Part model, mm, in its own coordinate system. Face numbers are marked on the shaded views. A direction names the side the tool comes from. Coordinates: 2 decimals unless noted, no trailing zeros. Loops run counter-clockwise (first coordinate to the right, second up) from the corner with the lowest first, then second, coordinate; pieces in that order, holes last. Notation, with made-up numbers: (88.25, 59.5) -> (134.25, 59.5) arc R23 ccw to (134.25, 87.5) -> close; hole circle Ø5 at (32.25, 29). An arc over 180 degrees is marked (long way). One line per question, with ' | ' between items. Start each with the question number.
1) Cut at C-C (y = -0.5). List the corners of the cut face in (x, z) (3 decimals), plus the area to 3 significant figures.
2) 3-axis set-ups, long thin cutter, end or side, ignore diameter. For the marked faces 4, 5, 6 and 7: which of +Z, -Z, +X, -X, +Y, -Y reach the whole face in a straight line?
3) Two-plate mould, pull along X, no slides. Class the marked faces 1, 2 and 3: released by +X, released by -X, zero draft, split by the parting line, or undercut.
4) Cut at D-D (z = 0.8). List the corners of the cut face in (x, y) (3 decimals), plus the area to 3 significant figures.
5) Drop flat-ended pins along their axis: pin 1 (1.2 mm diameter, centred on x = -3.5, y = 0, fed in from +Z); pin 2 (1.4 mm diameter, centred on x = -7, z = -0.5, fed in from -Y); pin 3 (1.4 mm diameter, centred on x = -7, z = -0.5, fed in from +Y). Give the stop position or say it passes through.
6) Cut at B-B (y = 1.1). List the corners of the cut face in (x, z) (3 decimals), plus the area to 3 significant figures.
7) Cut at A-A (x = 0). List the corners of the cut face in (y, z) (3 decimals), plus the area to 3 significant figures.
8) Probe L1, parallel to Z at x = 0, y = -0.7; L2, parallel to Y at x = -7.5, z = -0.35; L3, parallel to Z at x = -3.25, y = -0.6. List the from-to ranges inside material, lowest first. Write a range as from..to.
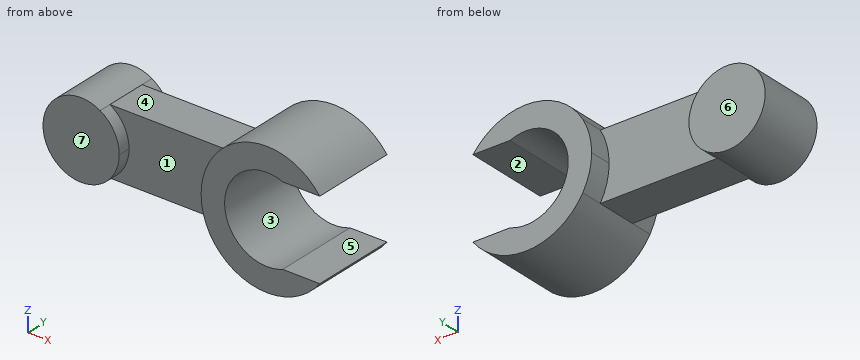
from build123d import *

# Parameters (mm, degrees)
F1_DEPTH = 1.23
F2_DEPTH = 0.765
F3_DEPTH = 1.595
F4_DEPTH = 1.595
F5_DEPTH = 0.765
F6_DEPTH = 1.23


with BuildPart() as f1:
    # F0 (on Front) → F1 (new body)
    with BuildSketch(Plane.XZ):
        with BuildLine():
            ThreePointArc((-6.54775, -1.24), (-6.022378, -0.716374), (-5.83, 0))
            ThreePointArc((-5.83, 0), (-6.022378, 0.716374), (-6.54775, 1.24))
            ThreePointArc((-6.54775, 1.24), (-8.69, 0), (-6.54775, -1.24))
        make_face()
    extrude(amount=F1_DEPTH)

    # F0 (on Front) → F2 (join)
    with BuildSketch(Plane.XZ):
        with BuildLine():
            Line((-5.83, 0), (-5.83, 1.24))
            Line((-5.83, 1.24), (-6.54775, 1.24))
            ThreePointArc((-6.54775, 1.24), (-6.022378, 0.716374), (-5.83, 0))
        make_face()
        with BuildLine():
            Line((-6.54775, -1.24), (-5.83, -1.24))
            Line((-5.83, -1.24), (-5.83, 0))
            ThreePointArc((-5.83, 0), (-6.022378, -0.716374), (-6.54775, -1.24))
        make_face()
        with BuildLine():
            ThreePointArc((-2.47, 0), (-2.385088, 0.642073), (-2.136188, 1.24))
            Line((-2.136188, 1.24), (-5.83, 1.24))
            Line((-5.83, 1.24), (-5.83, 0))
            Line((-5.83, 0), (-2.47, 0))
        make_face()
        with BuildLine():
            Line((-5.83, -1.24), (-2.136188, -1.24))
            ThreePointArc((-2.136188, -1.24), (-2.385088, -0.642073), (-2.47, 0))
            Line((-2.47, 0), (-5.83, 0))
            Line((-5.83, 0), (-5.83, -1.24))
        make_face()
    extrude(amount=F2_DEPTH)

    # F0 (on Front) → F3 (join)
    with BuildSketch(Plane.XZ):
        with BuildLine():
            Line((1.7075, 1.475), (1.981231, 1.475))
            ThreePointArc((1.981231, 1.475), (-0.140745, 2.465987), (-2.136188, 1.24))
            ThreePointArc((-2.136188, 1.24), (-2.385088, 0.642073), (-2.47, 0))
            ThreePointArc((-2.47, 0), (-2.385088, -0.642073), (-2.136188, -1.24))
            ThreePointArc((-2.136188, -1.24), (-0.140745, -2.465987), (1.981231, -1.475))
            Line((1.981231, -1.475), (1.7075, -1.475))
            Line((1.7075, -1.475), (0.593696, -1.475))
            ThreePointArc((0.593696, -1.475), (-1.59, 0), (0.593696, 1.475))
            Line((0.593696, 1.475), (1.7075, 1.475))
        make_face()
    extrude(amount=F3_DEPTH)

    # F0 (on Front) → F4 (join)
    with BuildSketch(Plane.XZ):
        with BuildLine():
            Line((1.7075, 1.475), (1.981231, 1.475))
            ThreePointArc((1.981231, 1.475), (-0.140745, 2.465987), (-2.136188, 1.24))
            ThreePointArc((-2.136188, 1.24), (-2.385088, 0.642073), (-2.47, 0))
            ThreePointArc((-2.47, 0), (-2.385088, -0.642073), (-2.136188, -1.24))
            ThreePointArc((-2.136188, -1.24), (-0.140745, -2.465987), (1.981231, -1.475))
            Line((1.981231, -1.475), (1.7075, -1.475))
            Line((1.7075, -1.475), (0.593696, -1.475))
            ThreePointArc((0.593696, -1.475), (-1.59, 0), (0.593696, 1.475))
            Line((0.593696, 1.475), (1.7075, 1.475))
        make_face()
    extrude(amount=-F4_DEPTH)

    # F0 (on Front) → F5 (join)
    with BuildSketch(Plane.XZ):
        with BuildLine():
            Line((-6.54775, -1.24), (-5.83, -1.24))
            Line((-5.83, -1.24), (-5.83, 0))
            ThreePointArc((-5.83, 0), (-6.022378, -0.716374), (-6.54775, -1.24))
        make_face()
        with BuildLine():
            Line((-5.83, 0), (-5.83, 1.24))
            Line((-5.83, 1.24), (-6.54775, 1.24))
            ThreePointArc((-6.54775, 1.24), (-6.022378, 0.716374), (-5.83, 0))
        make_face()
        with BuildLine():
            ThreePointArc((-2.47, 0), (-2.385088, 0.642073), (-2.136188, 1.24))
            Line((-2.136188, 1.24), (-5.83, 1.24))
            Line((-5.83, 1.24), (-5.83, 0))
            Line((-5.83, 0), (-2.47, 0))
        make_face()
        with BuildLine():
            Line((-5.83, -1.24), (-2.136188, -1.24))
            ThreePointArc((-2.136188, -1.24), (-2.385088, -0.642073), (-2.47, 0))
            Line((-2.47, 0), (-5.83, 0))
            Line((-5.83, 0), (-5.83, -1.24))
        make_face()
    extrude(amount=-F5_DEPTH)

    # F0 (on Front) → F6 (join)
    with BuildSketch(Plane.XZ):
        with BuildLine():
            ThreePointArc((-6.54775, -1.24), (-6.022378, -0.716374), (-5.83, 0))
            ThreePointArc((-5.83, 0), (-6.022378, 0.716374), (-6.54775, 1.24))
            ThreePointArc((-6.54775, 1.24), (-8.69, 0), (-6.54775, -1.24))
        make_face()
    extrude(amount=-F6_DEPTH)


solid = f1.part
Reported:
1) outline: (-6.548, -1.24) -> (-2.136, -1.24) arc R2.47 ccw to (1.981, -1.475) -> (0.594, -1.475) arc R1.59 cw (long way) to (0.594, 1.475) -> (1.981, 1.475) arc R2.47 ccw to (-2.136, 1.24) -> (-6.548, 1.24) arc R1.43 ccw (long way) to start | area: 23.8 mm²
2) face 4: +Z, +Y, -Y | face 5: +X, +Y, -Y | face 6: +Z, -Z, -X, +Y | face 7: +Z, -Z, -X, -Y
3) face 1: undercut | face 2: zero draft | face 3: undercut
4) outline: (-8.445, -1.23) -> (-6.075, -1.23) -> (-6.075, -0.765) -> (-2.337, -0.765) -> (-2.337, -1.595) -> (-1.374, -1.595) -> (-1.374, 1.595) -> (-2.337, 1.595) -> (-2.337, 0.765) -> (-6.075, 0.765) -> (-6.075, 1.23) -> (-8.445, 1.23) -> close | area: 14.6 mm²
5) pin 1: stops at z = 1.24 | pin 2: stops at y = -1.23 | pin 3: stops at y = 1.23
6) outline: circle Ø2.86 at (-7.26, 0); (-2.47, 0) arc R2.47 ccw to (-2.136, -1.24) arc R2.47 ccw to (1.981, -1.475) -> (0.594, -1.475) arc R1.59 cw (long way) to (0.594, 1.475) -> (1.981, 1.475) arc R2.47 ccw to (-2.136, 1.24) arc R2.47 ccw to start | area: 14.7 mm²
7) outline: (-1.595, -2.47) -> (1.595, -2.47) -> (1.595, -1.59) -> (-1.595, -1.59) -> close; (-1.595, 1.59) -> (1.595, 1.59) -> (1.595, 2.47) -> (-1.595, 2.47) -> close | area: 5.61 mm²
8) L1: z = -2.47..-1.59, 1.59..2.47 | L2: y = -1.23..1.23 | L3: z = -1.24..1.24
